from build123d import *

# Parameters (mm, degrees)
PAD_DEPTH       = 15
SKETCH002_R     = 67
POCKET_DEPTH    = 13.5
POCKET001_DEPTH = 13.5
PAD001_DEPTH    = 35
PAD002_DEPTH    = 35
SKETCH_R        = 9.5
POCKET002_DEPTH = 39.8207539141
SKETCH007_R     = 9.5
POCKET003_DEPTH = 97.217065943


with BuildPart() as part:
    # Sketch001 → Pad (new body)
    with BuildSketch(Plane.XY):
        with BuildLine():
            ThreePointArc((67.082039325, 20), (42.1720802134, 55.8705257759), (0.8477088241, 69.9948668814))
            Line((0.8477088241, 69.9948668814), (-65, 70.7923477994))
            ThreePointArc((-65, 70.7923477994), (-87.9606343369, 33.6277973957), (-44.3683356165, 30.7806886639))
            ThreePointArc((51.7489964992, 15.4285890907), (8.5170581243, 53.324100751), (-44.3683356165, 30.7806886639))
            ThreePointArc((51.7489964992, 15.4285890907), (61.7012261231, 10.0477638873), (67.082039325, 20))
        make_face()
    extrude(amount=PAD_DEPTH)

    # Sketch002 → Pocket (cut)
    with BuildSketch(Plane(origin=(0, 0, 0), x_dir=(1, 0, 0), z_dir=(0, 0, -1))):
        Circle(SKETCH002_R)
    extrude(amount=-POCKET_DEPTH, mode=Mode.SUBTRACT)

    # Sketch003 → Pocket001 (cut)
    with BuildSketch(Plane(origin=(0, 0, 0), x_dir=(1, 0, 0), z_dir=(0, 0, -1))):
        Polygon((-152.5343617943, -68.8522555402), (0.8113925418, -66.9950867015), (-35.4631, 35.7409), align=None)
    extrude(amount=-POCKET001_DEPTH, mode=Mode.SUBTRACT)

    # Sketch005 → Pad001 (new body)
    with BuildSketch(Plane.XY.offset(15)):
        Polygon((35.7520138156, 58.6156421796), (42.6985975202, 65.809040183), (64.2787915304, 44.9692890692), (57.3322078258, 37.7758910658), align=None)
    extrude(amount=-PAD001_DEPTH)

    # Sketch006 → Pad002 (new body)
    with BuildSketch(Plane.XY.offset(15)):
        Polygon((-40.5291145864, 67.4957611541), (-42.5812354464, 73.1339168789), (-14.3904568228, 83.3945211786), (-8.4624301934, 67.1074018724), align=None)
    extrude(amount=-PAD002_DEPTH)

    # Sketch → Pocket002 (cut, through all)
    with BuildSketch(Plane(origin=(46.5421108207, 48.1957666227, 0), x_dir=(0.7193398003, -0.6946583705, 0), z_dir=(-0.6946583705, -0.7193398003, 0))):
        with Locations((0, -20)):
            Circle(SKETCH_R)
    extrude(amount=-POCKET002_DEPTH, mode=Mode.SUBTRACT)

    # Sketch007 → Pocket003 (cut, through all)
    with BuildSketch(Plane(origin=(-28.4858461346, 78.2642190287, 0), x_dir=(-0.9396926208, -0.3420201433, 0), z_dir=(-0.3420201433, 0.9396926208, 0))):
        with Locations((0, -20)):
            Circle(SKETCH007_R)
    extrude(amount=-POCKET003_DEPTH, mode=Mode.SUBTRACT)


solid = part.part
The listing builds one solid part. Answer for the finished solid, in the listing's coordinates (mm). A direction names the side the tool comes from. Round coordinates to 2 decimals unless told otherwise and drop trailing zeros. Loops run counter-clockwise (first coordinate to the right, second up) from the corner with the lowest first, then second, coordinate; pieces in that order, holes last. Notation, with made-up numbers: M 22.25,55 L 66.25,55 A12 ccw 66.25,61 Z; hole C 39.5,19.5 d2. An arc over 180 degrees is marked long. Return JSON: item names as keys, results as strings.
Q1. Find the intervals of material crossed by line 1 along Z through (x, y) = (37, 45); line 2 along Y through (x, z) = (0.5, 11); line 3 along X through (y, z) = (70, -17.5), in increasing order. Write a range as from..to.
Results list:
{"line 1": "z = 13.5..15", "line 2": "y = 67..70", "line 3": "x = -41.44..-35.23, -15.72..-9.52"}
Q2. Find section B-B, the plane z = 9. Determine the outline of the cut face in (x, y), plus the area to 3 significant figures.
Results list:
{"outline": "M -77.03,67.94 L 0.81,67 A67 cw 65.76,12.84 A8 ccw 67.08,20 A70 ccw 58.29,38.76 L 64.28,44.97 L 42.7,65.81 L 36.71,59.6 A70 ccw 0.85,69.99 L -9.56,70.12 L -14.39,83.39 L -42.58,73.13 L -41.63,70.51 L -65,70.79 A25.49 ccw Z", "area": "976 mm2"}
Q3. Find section C-C, the plane x = 28.5. Determine the outline of the cut face in (y, z).
Results list:
{"outline": "M 45.87,13.5 L 60.64,13.5 L 60.64,0 L 63.94,0 L 63.94,15 L 45.87,15 Z"}
Q4. Find section D-D, the plane x = 3. Determine the outline of the cut face in (y, z).
Results list:
{"outline": "M 53.92,13.5 L 66.93,13.5 L 66.93,0 L 69.94,0 L 69.94,15 L 53.92,15 Z"}
Q5. The mould has two halves that part along Y. Classify faces 4 (the face through (19.74, 67.16, 7.4)), 5 (the face through (46.693, 48.05, -7.638)), 6 (the face through (60.85, 41.42, -2.25)): released by +Y, released by -Y, zero draft, split by the parting line, or undercut.
Results list:
{"face 4": "released by +Y", "face 5": "released by -Y", "face 6": "undercut"}
Q6. Find section A-A, the plane z = -5.5. Determine the outline of the cut face in (x, y).
Results list:
{"outline": "M -42.58,73.13 L -40.53,67.5 L -8.46,67.11 L -14.39,83.39 Z; M 35.75,58.62 L 57.33,37.78 L 64.28,44.97 L 42.7,65.81 Z"}
Q7. Which of the six approach directions +Z, -Z, +X, -X, +Y, -Y give full straight-line access (tool end or side, diameter ignored) to faces 1 (the face through (-28.683, 78.192, -2.255)), 2 (the face through (63.444, 29.578, 7.395)), 3 (the face through (42.41, 51.87, 6.66))?
Results list:
{"face 1": "+Z, -Z, -X, +Y", "face 2": "+Z, -Z, +X", "face 3": "-Z, -X, -Y"}
Q8. Each of these flat-tipped pins is pushed along its axis until it touches: pin 1 Ø8 at (x, z) = (-24.5, 10.5) entering from +Y; pin 2 Ø17.5 at (x, y) = (-9.5, 51) entering from -Z; pin 3 Ø3 at (x, z) = (-38.5, 9) entering from +Y; pin 4 Ø23 at (x, y) = (53, 38.5) entering from -Z. Where does it stop, or does it pass through?
Results list:
{"pin 1": "stops at y = 81.17", "pin 2": "stops at z = 13.5", "pin 3": "stops at y = 75.17", "pin 4": "stops at z = -20"}
